Autodesk Inventor part; units mm, degrees
ref_plane "YZ Plane" through (0, 0, 0) normal (1, 0, 0) x (0, 1, 0)
ref_plane "XZ Plane" through (0, 0, 0) normal (0, 1, 0) x (-1, 0, 0)
ref_plane "XY Plane" through (0, 0, 0) normal (0, 0, 1) x (1, 0, 0)
sketch "Boceto1" plane through (0, 0, 0) normal (0, 1, 0) x (-1, 0, 0)
  line L0 (25, 11) -> (-25, 11)
  line L1 (-25, 11) -> (-25, -11)
  line L2 (-25, -11) -> (25, -11)
  line L3 (25, -11) -> (25, 11)
  point P0 (0, 0)
  dimension "largo" = 50
  dimension "ancho" = 22
  dimension "d2" = 11
  dimension "d3" = 25
extrude "Extrusión1" add sketch "Boceto1" along normal blind 1
sketch "Boceto2" plane through (0, 1, 0) normal (0, 1, 0) x (1, 0, 0)
  line L0 (-25, 11) -> (-25, -11)
  line L1 (-25, 7) -> (-15, 7)
  line L2 (-15, 7) -> (-15, 11)
  line L3 (-15, 11) -> (-25, 11)
  line L4 (-25, 11) -> (-25, 7)
  line L5 (-11, 11) -> (-1, 11)
  line L6 (-1, 11) -> (-1, 7)
  line L7 (-1, 7) -> (-11, 7)
  line L8 (-11, 7) -> (-11, 11)
  line L9 (25, 11) -> (-25, 11)
  line L10 (3, 11) -> (13, 11)
  line L11 (13, 11) -> (13, 7)
  line L12 (13, 7) -> (3, 7)
  line L13 (3, 7) -> (3, 11)
  line L14 (18.5, 11) -> (25, 11)
  line L15 (25, 11) -> (25, 7)
  line L16 (25, 7) -> (18.5, 7)
  line L17 (18.5, 7) -> (18.5, 11)
  line L18 (25, -11) -> (25, 11)
  line L19 (25, -3.5465) -> (22, -3.5465)
  line L20 (22, -3.5465) -> (22, -1.5465)
  line L21 (22, -1.5465) -> (25, -1.5465)
  line L22 (25, -1.5465) -> (25, -3.5465)
  line L23 (25, -4.0465) -> (22, -4.0465)
  line L24 (22, -4.0465) -> (22, -6.0465)
  line L25 (22, -6.0465) -> (25, -6.0465)
  line L26 (25, -6.0465) -> (25, -4.0465)
  line L27 (25, -6.5465) -> (22, -6.5465)
  line L28 (22, -6.5465) -> (22, -8.5465)
  line L29 (22, -8.5465) -> (25, -8.5465)
  line L30 (25, -8.5465) -> (25, -6.5465)
  point P0 (0, 0)
  point P1 (25, -1.5465)
  point P2 (25, 11)
  point P3 (13, 11)
  dimension "d6" = 10
  dimension "d7" = 4
  dimension "d8" = 10
  dimension "d9" = 4
  dimension "d10" = 10
  dimension "d11" = 4
  dimension "d12" = 6.5
  dimension "d13" = 4
  dimension "d14" = 3
  dimension "d15" = 2
  dimension "d22" = 0
  dimension "d23" = 0
  dimension "d24" = 14
  dimension "d25" = 14
  dimension "d27" = 0
  dimension "d28" = 2
  dimension "d29" = 3
  dimension "d30" = 2
  dimension "d31" = 0.5
  dimension "d32" = 0.5
extrude "Extrusión2" add sketch "Boceto2" along normal blind 0.1
sketch "Boceto3" plane through (0, 1.1, 0) normal (0, 1, 0) x (1, 0, 0)
  circle A0 centre (-23, 9) radius 1.25
  circle A1 centre (-20, 9) radius 1.25
  circle A2 centre (-17, 9) radius 1.25
  line L0 (-15, 11) -> (-25, 11)
  line L1 (-25, 11) -> (-25, 7)
  line L2 (-25, 7) -> (-15, 7)
  circle A3 centre (-9, 9) radius 1.25
  circle A4 centre (-6, 9) radius 1.25
  circle A5 centre (-3, 9) radius 1.25
  line L3 (-11, 11) -> (-11, 7)
  circle A6 centre (5, 9) radius 1.25
  circle A7 centre (8, 9) radius 1.25
  circle A8 centre (11, 9) radius 1.25
  circle A9 centre (20.2, 9) radius 1.25
  circle A10 centre (23.2, 9) radius 1.25
  line L4 (18.5, 11) -> (18.5, 7)
  line L5 (3, 11) -> (3, 7)
  circle A11 centre (23.5, -7.5613) radius 0.75
  circle A12 centre (23.5, -5.1334) radius 0.75
  circle A13 centre (23.5, -2.4754) radius 0.75
  line L6 (22, -6.5465) -> (22, -8.5465)
  point P0 (0, 0)
  dimension "d33" = 2.5
  dimension "d34" = 2.5
  dimension "d35" = 2.5
  dimension "d36" = 2
  dimension "d37" = 2
  dimension "d38" = 3
  dimension "d39" = 2
  dimension "d40" = 3
  dimension "d41" = 2
  dimension "d42" = 2.5
  dimension "d43" = 2.5
  dimension "d44" = 2.5
  dimension "d45" = 3
  dimension "d46" = 3
  dimension "d47" = 2
  dimension "d48" = 2.5
  dimension "d49" = 2.5
  dimension "d50" = 2.5
  dimension "d51" = 3
  dimension "d52" = 3
  dimension "d53" = 2.5
  dimension "d54" = 2.5
  dimension "d56" = 3
  dimension "d58" = 1.7
  dimension "d59" = 2
  dimension "d60" = 1.5
  dimension "d61" = 1.5
  dimension "d62" = 1.5
  dimension "d63" = 1.5
extrude "Extrusión3" cut sketch "Boceto3" against normal blind 5.1
sketch "Boceto4" plane through (0, 1.1, 0) normal (0, 1, 0) x (1, 0, 0)
  circle A0 centre (-20, 9) radius 1.25
sketch "Boceto5" plane through (0, 1.1, 0) normal (0, 1, 0) x (1, 0, 0)
  circle A0 centre (-6, 9) radius 1.25
sketch "Boceto6" plane through (0, 1.1, 0) normal (0, 1, 0) x (1, 0, 0)
  circle A0 centre (8, 9) radius 1.25
sketch "Boceto7" plane through (0, 1.1, 0) normal (0, 1, 0) x (1, 0, 0)
  circle A0 centre (20.2, 9) radius 1.25
sketch "Boceto8" plane through (0, 1.1, 0) normal (0, 1, 0) x (1, 0, 0)
  circle A0 centre (23.5, -2.4754) radius 0.75
sketch "Boceto9" plane through (0, 1.1, 0) normal (0, 1, 0) x (1, 0, 0)
  circle A0 centre (23.5, -5.1334) radius 0.75
sketch "Boceto10" plane through (0, 1.1, 0) normal (0, 1, 0) x (1, 0, 0)
  circle A0 centre (23.5, -7.5613) radius 0.75
properties part number "CARGADOR BATERIA LIPO LITIO 4 CELDAS 5A 18650"
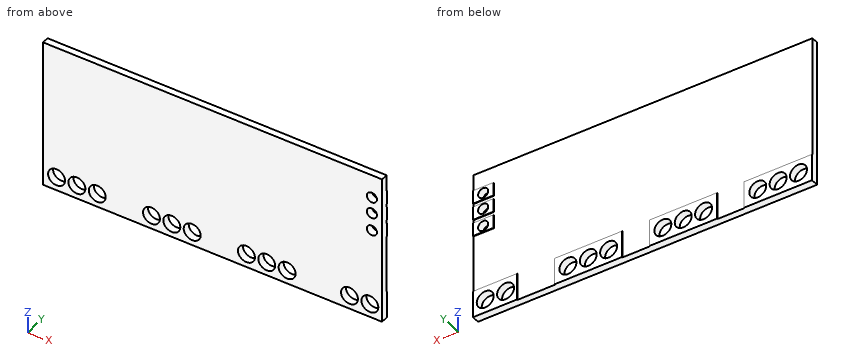
Read the model definition and answer for the solid it produces. Units are mm, in the model's axes. Round coordinates to 2 decimals unless told otherwise and drop trailing zeros. Write each loop counter-clockwise with the first axis right and the second up, starting at its lowest first coordinate (ties: lowest second). Pieces come first, ordered by that corner, then holes.
1. Given pin 1 Ø1.5 at (x, z) = (11, -9) entering from +Y; pin 2 Ø3 at (x, z) = (-17, -9) entering from -Y; pin 3 Ø5 at (x, z) = (-11.5, 8.5) entering from +Y, each flat-ended and moving along its own axis, determine where each tip first touches the part or whether it passes through.
2. The part is cut by section A-A, the plane x = -23. Determine the outline of the cut face in (y, z).
3. Straight lines are drawn through the part: L1, parallel to Z at x = -17, y = 0.6; L2, parallel to Y at x = -10, z = 1; L3, parallel to Z at x = -10, y = 0.1. For each, find the intervals that lie inside material, in ascending order.
4. The part is cut by section B-B, the plane z = -9. State how many separate pieces and enclosed holes the cut face has, then the cut area to 3 significant figures.
Values:
1. pin 1: passes through
1. pin 2: stops at y = 0
1. pin 3: stops at y = 1
2. outline: (0, -11) - (1.1, -11) - (1.1, -10.25) - (0, -10.25) - close; (0, -7.75) - (1.1, -7.75) - (1.1, -7) - (1, -7) - (1, 11) - (0, 11) - close
3. L1: z = -11 to -10.25, -7.75 to 11
3. L2: y = 0 to 1
3. L3: z = -11 to -9.75, -8.25 to 11
4. separate pieces: 12
4. enclosed holes: 0
4. area: 23.4 mm2
